Geometry check sheet. Reference: drawing and pictorial views, mm from the part's lowest x, y, z. Coordinates: 2 decimals unless noted, no trailing zeros. Write each loop counter-clockwise with the first axis right and the second up, starting at its lowest first coordinate (ties: lowest second). Pieces come first, ordered by that corner, then holes. Notation, with made-up numbers: (17, 0) - (32, 0) arc R24 ccw to (32, 31) - close; hole circle Ø1 at (72, -24). An arc over 180 degrees is marked (long way). Answer as a JSON object with one key per item and string values. Group by question number.
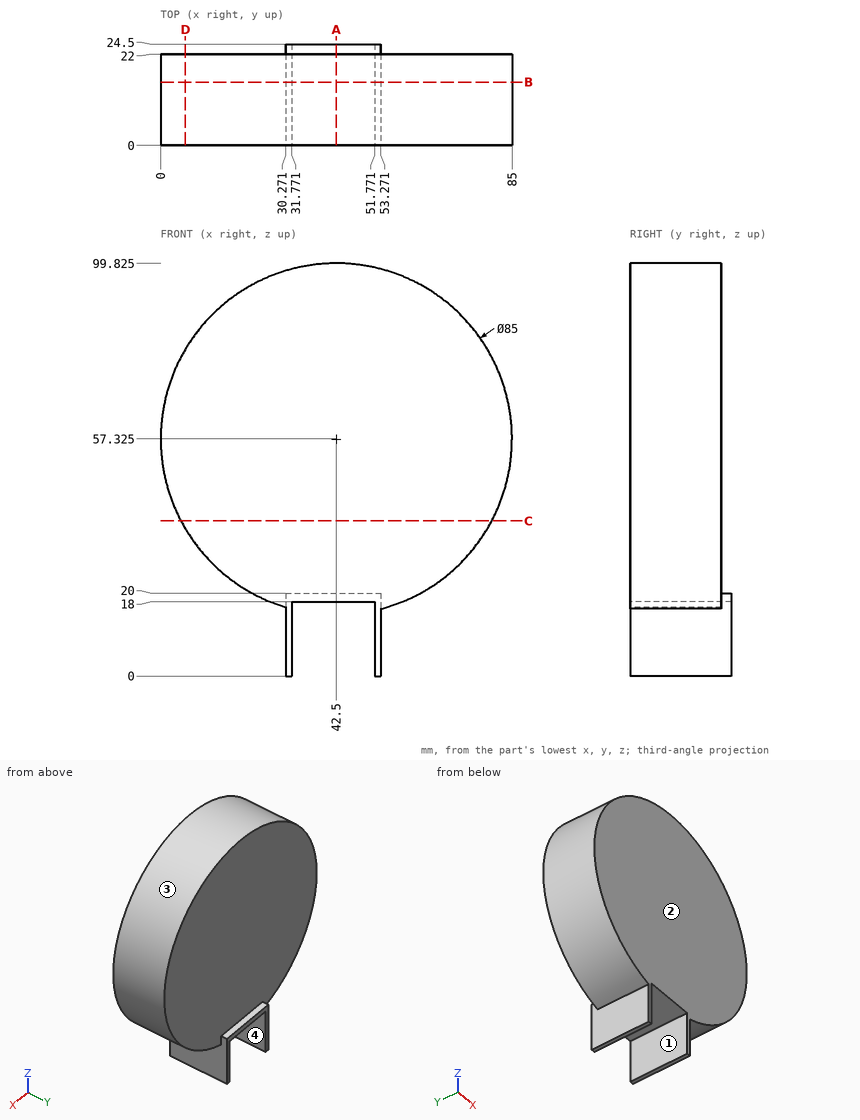
(1) Section check C-C (z = 37.5). Record the cut outline in (x, y), and give its area (3 significant figures).
(2) Draft check along X on the marked faces 1, 2, 3 and 4. Enter one of: +X half, -X half, draft (parallel to the pull), parting line (faces both ways), or undercut.
(3) Section check B-B (y = 15.25). Record the cut outline in (x, z) (1 decimal), and give its area (3 significant figures).
(4) Gauge pin test, flat ends, axial feed: pin 1 (5 mm diameter, centred on x = 64.5, y = 18, fed in from -Z); pin 2 (6 mm diameter, centred on x = 75.5, y = 14.5, fed in from -Z); pin 3 (0.8 mm diameter, centred on x = 40, y = 23, fed in from +Z). Record the tip position at first contact, or that the pin passes through.
(5) Section check A-A (x = 42.5). Record the cut outline in (y, z) (1 decimal).
(6) Section check D-D (x = 6). Record the cut outline in (y, z).
(7) Material ranges on L1, parallel to X at y = 9.75, z = 5.5; L2, parallel to Y at x = 60, z = 91; L3, parallel to X at y = 13, z = 47, recorded low to high. Write a range as [from, to].
Conclusion:
{
 "1": {"outline": "(4.91, 0) - (80.09, 0) - (80.09, 22) - (4.91, 22) - close", "area": "1,650 mm^2"},
 "2": {"face 1": "undercut", "face 2": "draft", "face 3": "parting line", "face 4": "undercut"},
 "3": {"outline": "(30.3, 0) - (31.8, 0) - (31.8, 18) - (51.8, 18) - (51.8, 0) - (53.3, 0) - (53.3, 16.2) arc R42.5 ccw (long way) to (30.3, 16.6) - close", "area": "5,670 mm^2"},
 "4": {"pin 1": "stops at z = 19.56", "pin 2": "stops at z = 27.22", "pin 3": "stops at z = 20"},
 "5": {"outline": "(0, 18) - (24.5, 18) - (24.5, 20) - (22, 20) - (22, 99.8) - (0, 99.8) - close"},
 "6": {"outline": "(0, 35.55) - (22, 35.55) - (22, 79.1) - (0, 79.1) - close"},
 "7": {"L1": "x = [30.27, 31.77], [51.77, 53.27]", "L2": "y = [0, 22]", "L3": "x = [1.27, 83.73]"}
}
